```python
from build123d import *

# Parameters (mm, degrees)
F0_R     = 2.5
F1_DEPTH = 50
F2_R     = 25
F3_DEPTH = 25
F4_DEPTH = 50
F5_DEPTH = 25
F6_R     = 27.1
F6_R_2   = 25.9
F7_DEPTH = 5
F8_DEPTH = 25


# Not quite as in the source:
# - a feature names something its author has since deleted; it is built from what else it names


with BuildPart() as f1:
    # F0 (on Front) → F1 (new body)
    with BuildSketch(Plane.XZ):
        Polygon((90, 4.9383143896), (0, 4.9383143896), (0, -0.0616856104), (0, -3.0616856104), (90, -3.0616856104), (90, -0.0616856104), align=None)
        with BuildLine():
            Line((0, -0.0616856104), (0, 4.9383143896))
            Line((0, 4.9383143896), (-14, 4.9383143896))
            Line((-14, 4.9383143896), (-14, -3.0616856104))
            ThreePointArc((-14, -3.0616856104), (-7, -10.0616856104), (0, -3.0616856104))
            Line((0, -3.0616856104), (0, -0.0616856104))
        make_face()
        with Locations((-7, 0)):
            Circle(F0_R, mode=Mode.SUBTRACT)
    extrude(amount=F1_DEPTH)

    # F2 (on Top) → F3 (cut)
    with BuildSketch(Plane.XY):
        with Locations((45, -50)):
            Circle(F2_R)
    extrude(amount=-F3_DEPTH, mode=Mode.SUBTRACT)

    # F0 (on Front) → F4 (join)
    with BuildSketch(Plane.XZ):
        Polygon((90, 4.9383143896), (0, 4.9383143896), (0, -0.0616856104), (0, -3.0616856104), (90, -3.0616856104), (90, -0.0616856104), align=None)
        with BuildLine():
            Line((0, -0.0616856104), (0, 4.9383143896))
            Line((0, 4.9383143896), (-14, 4.9383143896))
            Line((-14, 4.9383143896), (-14, -3.0616856104))
            ThreePointArc((-14, -3.0616856104), (-7, -10.0616856104), (0, -3.0616856104))
            Line((0, -3.0616856104), (0, -0.0616856104))
        make_face()
        with Locations((-7, 0)):
            Circle(F0_R, mode=Mode.SUBTRACT)
        with BuildLine():
            Line((104, 4.9383143896), (90, 4.9383143896))
            Line((90, 4.9383143896), (90, -0.0616856104))
            Line((90, -0.0616856104), (90, -3.0616856104))
            ThreePointArc((90, -3.0616856104), (97, -10.0616856104), (104, -3.0616856104))
            Line((104, -3.0616856104), (104, -0.0616856104))
            Line((104, -0.0616856104), (104, 4.9383143896))
        make_face()
        with Locations((97, -0.0616856104)):
            Circle(F0_R, mode=Mode.SUBTRACT)
    extrude(amount=F4_DEPTH)

    # F2 (on Top) → F5 (cut)
    with BuildSketch(Plane.XY):
        with Locations((45, -50)):
            Circle(F2_R)
    extrude(amount=-F5_DEPTH, mode=Mode.SUBTRACT)

    # F6 (on Top) → F7 (cut)
    with BuildSketch(Plane.XY):
        with Locations((45, -50)):
            Circle(F6_R)
        with Locations((45, -50)):
            Circle(F6_R_2, mode=Mode.SUBTRACT)
    extrude(amount=F7_DEPTH, mode=Mode.SUBTRACT)

    # F2 (on Top) → F8 (cut)
    with BuildSketch(Plane.XY):
        with Locations((45, -50)):
            Circle(F2_R)
    extrude(amount=F8_DEPTH, mode=Mode.SUBTRACT)


solid = f1.part
```
Model file for the job. Use its own axes, mm. A direction names the side the tool comes from. Give positions to 0.01 mm unless a question says otherwise; leave off trailing zeros. Loops run counter-clockwise (first coordinate to the right, second up) from the corner with the lowest first, then second, coordinate; pieces in that order, holes last. Notation, with made-up numbers: (23, 50.5) -> (66, 50.5) arc R19 ccw to (66, 70.5) -> close; hole circle Ø2 at (6, 16). An arc over 180 degrees is marked (long way). Write each question's results on one line, items separated by ' | '.
(1) Cut at A-A on x = -7. List the corners of the cut face in (y, z).
Geometry results:
outline: (-50, -10.06) -> (0, -10.06) -> (0, -2.5) -> (-50, -2.5) -> close; (-50, 2.5) -> (0, 2.5) -> (0, 4.94) -> (-50, 4.94) -> close
(2) Probe line 1 along Z through (x, y) = (-7, -24); line 2 along Z through (x, y) = (97, -26); line 3 along X through (y, z) = (-13, 1.75). List the from-to ranges inside material, lowest first.
Geometry results:
line 1: z = -10.06 to -2.5, 2.5 to 4.94 | line 2: z = -10.06 to -2.56, 2.44 to 4.94 | line 3: x = -14 to -8.79, -5.21 to 95.28, 98.72 to 104
(3) Cut at C-C on y = -26.5. List the corners of the cut face in (x, z).
Geometry results:
outline: (-14, -3.06) arc R7 ccw to (0, -3.06) -> (36.47, -3.06) -> (36.47, 4.94) -> (34.11, 4.94) -> (34.11, 0) -> (31.5, 0) -> (31.5, 4.94) -> (-14, 4.94) -> close; (53.53, -3.06) -> (90, -3.06) arc R7 ccw to (104, -3.06) -> (104, 4.94) -> (58.5, 4.94) -> (58.5, 0) -> (55.89, 0) -> (55.89, 4.94) -> (53.53, 4.94) -> close; hole circle Ø5 at (-7, 0); hole circle Ø5 at (97, -0.06)
(4) Cut at D-D on y = -10.5. List the corners of the cut face in (x, z), and give its area (3 significant figures).
Geometry results:
outline: (-14, -3.06) arc R7 ccw to (0, -3.06) -> (90, -3.06) arc R7 ccw to (104, -3.06) -> (104, 4.94) -> (-14, 4.94) -> close; hole circle Ø5 at (-7, 0); hole circle Ø5 at (97, -0.06) | area: 1,060 mm²
(5) Flat gauge pins, fed straight in: pin 1 Ø6 at (x, z) = (56, -5.5) entering from -Y; pin 2 Ø25 at (x, y) = (55.5, -23) entering from -Z; pin 3 Ø8 at (x, z) = (-7, 0) entering from +Y; pin 4 Ø2 at (y, z) = (-19.5, -8) entering from +X. Where does each tip first touch, or does it go through?
Geometry results:
pin 1: stops at y = -28.49 | pin 2: stops at z = -3.06 | pin 3: stops at y = 0 | pin 4: stops at x = 102.79
(6) Pull direction X, two halves, no side cores. Call faces 1 (the flat face through (104, -25, 1)), 2 (the cylindrical face through (96.85, -24.65, -10.06)), 3 (the flat face through (46, -19, 4.938)): released by +X, released by -X, zero draft, split by the parting line, or undercut.
Geometry results:
face 1: released by +X | face 2: undercut | face 3: zero draft
(7) Tool access for faces 4 (the flat face through (3, -50, -1)), 5 (the flat face through (44, -19, -3.062)), 6 (the flat face through (41, -24, 0)): list every direction of +Z, -Z, +X, -X, +Y, -Y with a clear straight run to the whole face (end or side of a thin tool).
Geometry results:
face 4: +Z, -Z, +X, -X, -Y | face 5: -Z, +Y, -Y | face 6: +Z
(8) Cut at B-B on z = -6. List the corners of the cut face in (x, y), and give its area (3 significant figures).
Geometry results:
outline: (-13.35, -50) -> (-0.65, -50) -> (-0.65, 0) -> (-13.35, 0) -> close; (90.65, -50) -> (103.35, -50) -> (103.35, 0) -> (90.65, 0) -> close | area: 1,270 mm²
